Read the model definition and answer for the solid it produces. Units are mm, in the model's axes. A direction names the side the tool comes from. Coordinates: 2 decimals unless noted, no trailing zeros. Loops run counter-clockwise (first coordinate to the right, second up) from the corner with the lowest first, then second, coordinate; pieces in that order, holes last.
from build123d import *

# Parameters (mm, degrees)
BOSS_EXTRUDE1_DEPTH = 8.89
CUT_EXTRUDE2_DEPTH  = 8.89
FILLET1_R           = 8.89
SKETCH4_R           = 25.4
SKETCH11_R          = 15.875
SKETCH12_R          = 9.525
CUT_EXTRUDE3_DEPTH  = 25.13


with BuildPart() as part:
    # Sketch1 → Boss-Extrude1 (new body)
    with BuildSketch(Plane(origin=(0, 0, 0), x_dir=(1, 0, 0), z_dir=(0, 1, 0))):
        with BuildLine():
            Line((0, 0), (63.5, 0))
            Line((63.5, 0), (63.5, 50.8))
            Line((63.5, 50.8), (0, 50.8))
            ThreePointArc((0, 50.8), (-25.4, 25.4), (0, 0))
        make_face()
    extrude(amount=BOSS_EXTRUDE1_DEPTH)

    # Sketch2 → Cut-Extrude2 (cut)
    with BuildSketch(Plane(origin=(0, 8.89, 0), x_dir=(1, 0, 0), z_dir=(0, 1, 0))):
        with BuildLine():
            Line((41.91, 34.925), (41.91, 15.875))
            ThreePointArc((41.91, 15.875), (48.26, 9.525), (54.61, 15.875))
            Line((54.61, 15.875), (54.61, 34.925))
            ThreePointArc((54.61, 34.925), (48.26, 41.275), (41.91, 34.925))
        make_face()
    extrude(amount=-CUT_EXTRUDE2_DEPTH, mode=Mode.SUBTRACT)

    # Fillet1
    fillet1_edges = [part.edges().sort_by_distance(p)[0] for p in [
        (63.5, 4.445, -50.8),
        (63.5, 4.445, 0),
    ]]
    fillet(fillet1_edges, radius=FILLET1_R)

    # Sketch4 → Loft2 section 0
    with BuildSketch(Plane(origin=(0, 8.89, 0), x_dir=(1, 0, 0), z_dir=(0, 1, 0))):
        with Locations((0, 25.4)):
            Circle(SKETCH4_R)
    # Sketch11 → Loft2 section 1
    with BuildSketch(Plane(origin=(0, 24.13, 0), x_dir=(1, 0, 0), z_dir=(0, 1, 0))):
        with Locations((0, 25.4)):
            Circle(SKETCH11_R)
    loft()

    # Sketch12 → Cut-Extrude3 (cut, through all)
    with BuildSketch(Plane(origin=(0, 24.13, 0), x_dir=(1, 0, 0), z_dir=(0, 1, 0))):
        with Locations(Location((0, 25.4, 0), (0, 0, 270))):  # turned: the seam where the file's is
            Circle(SKETCH12_R)
    extrude(amount=-CUT_EXTRUDE3_DEPTH, mode=Mode.SUBTRACT)


solid = part.part
Q1. A cutting plane is placed at A-A (x = 48.26). Give the vertices of the cut face in (y, z) (3 decimals).
Findings below:
outline: (0, -50.8) - (8.89, -50.8) - (8.89, -41.275) - (0, -41.275) - close; (0, -9.525) - (8.89, -9.525) - (8.89, 0) - (0, 0) - close
Q2. A cutting plane is placed at C-C (z = -20). Count the separate pieces of the cut face and the enclosed holes in it, then the cut area to 3 significant figures.
Findings below:
separate pieces: 3
enclosed holes: 0
area: 900 mm2
Q3. A cutting plane is placed at B-B (y = 5.25). Give the vertices of the cut face in (x, z) (3 decimals).
Findings below:
outline: (0, -50.8) - (54.61, -50.8) arc R8.89 ccw to (63.5, -41.91) - (63.5, -8.89) arc R8.89 ccw to (54.61, 0) - (0, 0) arc R25.4 ccw to start; hole circle Ø19.05 at (0, -25.4); hole (41.91, -34.925) arc R6.35 ccw to (54.61, -34.925) - (54.61, -15.875) arc R6.35 ccw to (41.91, -15.875) - close
Q4. Which of the six approach directions +Z, -Z, +X, -X, +Y, -Y give full straight-line access (tool end or side, diameter ignored) to faces 5 (the face through (-25.394, 4.383, -25.959)), 6 (the face through (41.91, 5, -26))?
Findings below:
face 5: -X, +Y, -Y
face 6: +Y, -Y
Q5. Straight lines are drawn through the part: probe 1 along X at (y, z) = (7.25, -25.4) (3 decimals); probe 2 along X at (y, z) = (6.75, -21); probe 3 along X at (y, z) = (22.25, -28). For each, find the intervals that lie inside material, in ascending order.
Findings below:
probe 1: x = -25.4 to -9.525, 9.525 to 41.91, 54.61 to 63.5
probe 2: x = -25.02 to -8.45, 8.45 to 41.91, 54.61 to 63.5
probe 3: x = -16.85 to -9.16, 9.16 to 16.85
Q6. Flat-ended cylindrical pins translate along their axes: pin 1 Ø15 at (x, z) = (0, -25.4) entering from -Y; pin 2 Ø1 at (y, z) = (8, -43.5) entering from -X; pin 3 Ø2 at (y, z) = (18.5, -9) entering from +X; pin 4 Ø3 at (x, z) = (-16, -10.5) entering from -Y. Find the tip coordinate at first contact, or state that the pin passes through.
Findings below:
pin 1: passes through
pin 2: stops at x = -18.31
pin 3: stops at x = 12.14
pin 4: stops at y = 0
Q7. A cutting plane is placed at D-D (y = 10.25). Give the vertices of the cut face in (x, z) (3 decimals).
Findings below:
outline: circle Ø49.1 at (0, -25.4); hole circle Ø19.05 at (0, -25.4)
Q8. Determine the mould class of faces 1 (the face through (60.83, 4.51, -2.54)), 2 (the face through (2.861, 12.234, -16.315)), 3 (the face through (48.4, 4.507, -41.273)), 4 (the face through (0, 24.13, -15)) for opening direction X: +X half, -X half, draft (parallel to the pull), parting line (faces both ways), or undercut.
Findings below:
face 1: +X half
face 2: undercut
face 3: undercut
face 4: draft
